```python
from build123d import *

# Parameters (mm, degrees)
SKICA1_R                 = 2
P_IDAT_VYSUNUT_M3_DEPTH  = 2
ODEBRAT_START            = -18
SKICA5_R                 = 2.5
SKICA5_R_2               = 2
ODEBRAT_VYSUNUT_M1_DEPTH = 18
SKICA1_6_R               = 2
ODEBRAT_VYSUNUT_M3_DEPTH = 1


with BuildPart() as part:
    # Skica1 → P_idat vysunut_m3 (new body)
    # profile 1 of 2: a face of its own
    with BuildSketch(Plane(origin=(0, 0, 0), x_dir=(1, 0, 0), z_dir=(0, 1, 0))):
        with BuildLine():
            Line((108.040914438, 105.971068272), (106.006427981, 34.226677149))
            ThreePointArc((106.006427981, 34.226677149), (110.004588085, 37.999997369), (113.994081517, 34.217515135))
            Line((113.994081517, 34.217515135), (112.040914438, 106))
            Line((112.040914438, 106), (110, 111.642221926))
            Line((110, 111.642221926), (108.040914438, 105.971068272))
        make_face()
    # profile 2 of 2: a face of its own
    with BuildSketch(Plane(origin=(0, 0, 0), x_dir=(1, 0, 0), z_dir=(0, 1, 0))):
        with BuildLine():
            ThreePointArc((106, 34), (107.171572875, 31.171572875), (110, 30))
            ThreePointArc((110, 30), (112.828427125, 31.171572875), (114, 34))
            Line((114, 34), (113.994081517, 34.217515135))
            ThreePointArc((113.994081517, 34.217515135), (110.004588085, 37.999997369), (106.006427981, 34.226677149))
            Line((106.006427981, 34.226677149), (106, 34))
        make_face()
        with Locations(Location((110, 34, 0), (0, 0, 270))):
            Circle(SKICA1_R, mode=Mode.SUBTRACT)
    extrude(amount=P_IDAT_VYSUNUT_M3_DEPTH)

    # Skica5 → Odebrat vysunut_m1 (cut)
    with BuildSketch(Plane(origin=(0, 2, 0), x_dir=(1, 0, 0), z_dir=(0, 1, 0)).offset(ODEBRAT_START)):
        with Locations(Location((110, 34, 0), (0, 0, 270))):
            Circle(SKICA5_R)
        with Locations((110, 34)):
            Circle(SKICA5_R_2, mode=Mode.SUBTRACT)
    extrude(amount=ODEBRAT_VYSUNUT_M1_DEPTH, mode=Mode.SUBTRACT)

    # Skica1_6 → Odebrat vysunut_m3 (cut)
    # profile 1 of 2: a face of its own
    with BuildSketch(Plane(origin=(0, 0, 0), x_dir=(1, 0, 0), z_dir=(0, 1, 0))):
        with BuildLine():
            Line((108.040914438, 105.971068272), (106.006427981, 34.226677149))
            ThreePointArc((106.006427981, 34.226677149), (110.004588085, 37.999997369), (113.994081517, 34.217515135))
            Line((113.994081517, 34.217515135), (112.040914438, 106))
            Line((112.040914438, 106), (110, 111.642221926))
            Line((110, 111.642221926), (108.040914438, 105.971068272))
        make_face()
    # profile 2 of 2: a face of its own
    with BuildSketch(Plane(origin=(0, 0, 0), x_dir=(1, 0, 0), z_dir=(0, 1, 0))):
        with BuildLine():
            ThreePointArc((106, 34), (107.171572875, 31.171572875), (110, 30))
            ThreePointArc((110, 30), (112.828427125, 31.171572875), (114, 34))
            Line((114, 34), (113.994081517, 34.217515135))
            ThreePointArc((113.994081517, 34.217515135), (110.004588085, 37.999997369), (106.006427981, 34.226677149))
            Line((106.006427981, 34.226677149), (106, 34))
        make_face()
        with Locations((110, 34)):
            Circle(SKICA1_6_R, mode=Mode.SUBTRACT)
    extrude(amount=ODEBRAT_VYSUNUT_M3_DEPTH, mode=Mode.SUBTRACT)


solid = part.part
```
Can you work these out from the model? Positions are in its coordinate system, mm. Coordinates: 2 decimals unless noted, no trailing zeros. Loops run counter-clockwise (first coordinate to the right, second up) from the corner with the lowest first, then second, coordinate; pieces in that order, holes last.
Item 1: If we mould it in two halves opening along Z, with no side actions, what happens to faces 1 (the face through (110, 1, -71)), 2 (the face through (112.48, 1.49, -34.33)), 3 (the face through (109.034, 1.493, -108.846))? For each: released by +Z, released by -Z, zero draft, split by the parting line, or undercut.
Answers below:
face 1: zero draft
face 2: undercut
face 3: released by -Z
Item 2: Please list where these lines run through material, in increasing order: L1, parallel to X at y = 1.75, z = -34; L2, parallel to X at y = 1.65, z = -40.5; L3, parallel to X at y = 1.45, z = -85.5.
Answers below:
L1: x = 106 to 107.5, 112.5 to 114
L2: x = 106.18 to 113.82
L3: x = 107.46 to 112.6
Item 3: Suppose I cut it at C-C (z = -94). Please give me the cut outline in (x, y), then the cut area to 3 significant figures.
Answers below:
outline: (107.7, 1) - (112.37, 1) - (112.37, 2) - (107.7, 2) - close
area: 4.67 mm2
Item 4: Suppose I cut it at D-D (z = -43). Please give me the cut outline in (x, y), then the cut area to 3 significant figures.
Answers below:
outline: (106.26, 1) - (113.76, 1) - (113.76, 2) - (106.26, 2) - close
area: 7.50 mm2
Item 5: Suppose I cut it at B-B (x = 111). Please give me the cut outline in (y, z), then the cut area to 3 significant figures.
Answers below:
outline: (1, -108.88) - (2, -108.88) - (2, -36.29) - (1, -36.29) - close; (1, -31.71) - (2, -31.71) - (2, -30.13) - (1, -30.13) - close
area: 74.2 mm2
Item 6: Suppose I cut it at A-A (y = 1.45). Please give me the cut outline in (x, z).
Answers below:
outline: (106, -34) - (108.04, -105.97) - (110, -111.64) - (112.04, -106) - (114, -34) arc R4 ccw to start; hole circle Ø5 at (110, -34)
